Input: part model. Units: mm. Frame: model coordinates. Round coordinates to 2 decimals unless told otherwise and drop trailing zeros. Order: outer loops, then holes, each group sorted by start corner. A loop starts at its lowest first (then second) coordinate and runs counter-clockwise, first axis right, second up. Notation, with made-up numbers: (84.25, 51.5) -> (126.25, 51.5) arc R34 ccw to (126.25, 84.5) -> close; hole circle Ø10 at (-22.5, 49). An arc over 180 degrees is marked (long way). Use a Markdown table: item, result.
from build123d import *

# Parameters (mm, degrees)
SKETCH1_R           = 2.5
BOSS_EXTRUDE1_DEPTH = 5


with BuildPart() as part:
    # Sketch1 → Boss-Extrude1 (new body)
    with BuildSketch(Plane.XY):
        with BuildLine():
            Line((4.833962587, 7.00231299), (4.831156642, 7.163065475))
            Line((4.831156642, 7.163065475), (4.829008435, 7.286136175))
            Line((4.829008435, 7.286136175), (4.792643442, 9.369485213))
            Line((4.792643442, 9.369485213), (3.755980041, 9.831037496))
            Line((3.755980041, 9.831037496), (2.183417054, 8.464029347))
            Line((2.183417054, 8.464029347), (2.090520269, 8.383275404))
            Line((2.090520269, 8.383275404), (1.969180348, 8.27779622))
            ThreePointArc((1.969180348, 8.27779622), (1.769077823, 8.32285679), (1.567947285, 8.36308094))
            Line((1.567947285, 8.36308094), (1.5, 8.508794362))
            Line((1.5, 8.508794362), (1.447980152, 8.620351287))
            Line((1.447980152, 8.620351287), (0.567384684, 10.508794362))
            Line((0.567384684, 10.508794362), (-0.567384684, 10.508794362))
            Line((-0.567384684, 10.508794362), (-1.447980152, 8.620351287))
            Line((-1.447980152, 8.620351287), (-1.5, 8.508794362))
            Line((-1.5, 8.508794362), (-1.567947285, 8.36308094))
            ThreePointArc((-1.567947285, 8.36308094), (-1.769077823, 8.32285679), (-1.969180348, 8.27779622))
            Line((-1.969180348, 8.27779622), (-2.090520269, 8.383275404))
            Line((-2.090520269, 8.383275404), (-2.183417054, 8.464029347))
            Line((-2.183417054, 8.464029347), (-3.755980041, 9.831037496))
            Line((-3.755980041, 9.831037496), (-4.792643442, 9.369485213))
            Line((-4.792643442, 9.369485213), (-4.829008435, 7.286136175))
            Line((-4.829008435, 7.286136175), (-4.831156642, 7.163065475))
            Line((-4.831156642, 7.163065475), (-4.833962587, 7.00231299))
            ThreePointArc((-4.833962587, 7.00231299), (-5.001343841, 6.883759241), (-5.165818808, 6.761205332))
            Line((-5.165818808, 6.761205332), (-5.319570592, 6.808211969))
            Line((-5.319570592, 6.808211969), (-5.437281616, 6.844199841))
            Line((-5.437281616, 6.844199841), (-7.429901695, 7.453404935))
            Line((-7.429901695, 7.453404935), (-8.18921061, 6.610106952))
            Line((-8.18921061, 6.610106952), (-7.375057289, 4.692081926))
            Line((-7.375057289, 4.692081926), (-7.326962411, 4.578777493))
            Line((-7.326962411, 4.578777493), (-7.264141843, 4.430781509))
            ThreePointArc((-7.264141843, 4.430781509), (-7.368832073, 4.254397181), (-7.469240267, 4.075540618))
            Line((-7.469240267, 4.075540618), (-7.628818832, 4.055946834))
            Line((-7.628818832, 4.055946834), (-7.75099079, 4.040946004))
            Line((-7.75099079, 4.040946004), (-9.819125847, 3.787010949))
            Line((-9.819125847, 3.787010949), (-10.169788866, 2.707781148))
            Line((-10.169788866, 2.707781148), (-8.645891738, 1.286724086))
            Line((-8.645891738, 1.286724086), (-8.555869815, 1.202777285))
            Line((-8.555869815, 1.202777285), (-8.438284981, 1.093127654))
            ThreePointArc((-8.438284981, 1.093127654), (-8.462182296, 0.889411199), (-8.481162228, 0.685177906))
            Line((-8.481162228, 0.685177906), (-8.618974991, 0.602371644))
            Line((-8.618974991, 0.602371644), (-8.724483241, 0.538975892))
            Line((-8.724483241, 0.538975892), (-10.510533936, -0.534191634))
            Line((-10.510533936, -0.534191634), (-10.391918238, -1.662744616))
            Line((-10.391918238, -1.662744616), (-8.42177296, -2.341120038))
            Line((-8.42177296, -2.341120038), (-8.305389601, -2.381194042))
            Line((-8.305389601, -2.381194042), (-8.153371987, -2.433537904))
            ThreePointArc((-8.153371987, -2.433537904), (-8.092344324, -2.62936206), (-8.02661419, -2.82365829))
            Line((-8.02661419, -2.82365829), (-8.118832073, -2.955359075))
            Line((-8.118832073, -2.955359075), (-8.18943328, -3.056188048))
            Line((-8.18943328, -3.056188048), (-9.384575223, -4.763027631))
            Line((-9.384575223, -4.763027631), (-8.817190539, -5.745766731))
            Line((-8.817190539, -5.745766731), (-6.741453128, -5.564163239))
            Line((-6.741453128, -5.564163239), (-6.618832073, -5.553435287))
            Line((-6.618832073, -5.553435287), (-6.458666906, -5.53942265))
            ThreePointArc((-6.458666906, -5.53942265), (-6.323266501, -5.693494731), (-6.18419164, -5.844258315))
            Line((-6.18419164, -5.844258315), (-6.214869332, -6.002081362))
            Line((-6.214869332, -6.002081362), (-6.238355906, -6.12290931))
            Line((-6.238355906, -6.12290931), (-6.635938197, -8.16829288))
            Line((-6.635938197, -8.16829288), (-5.717890494, -8.835293579))
            Line((-5.717890494, -8.835293579), (-3.895474806, -7.825112067))
            Line((-3.895474806, -7.825112067), (-3.787818349, -7.765437119))
            Line((-3.787818349, -7.765437119), (-3.647199641, -7.687490896))
            ThreePointArc((-3.647199641, -7.687490896), (-3.460838455, -7.773170439), (-3.272466173, -7.854332985))
            Line((-3.272466173, -7.854332985), (-3.236299224, -8.010989254))
            Line((-3.236299224, -8.010989254), (-3.208610123, -8.130923927))
            Line((-3.208610123, -8.130923927), (-2.739887171, -10.161186083))
            Line((-2.739887171, -10.161186083), (-1.629915237, -10.397117901))
            Line((-1.629915237, -10.397117901), (-0.3759335, -8.73302793))
            Line((-0.3759335, -8.73302793), (-0.301856422, -8.634724327))
            Line((-0.301856422, -8.634724327), (-0.205098424, -8.506322127))
            ThreePointArc((-0.205098424, -8.506322127), (0, -8.508794362), (0.205098424, -8.506322127))
            Line((0.205098424, -8.506322127), (0.301856422, -8.634724327))
            Line((0.301856422, -8.634724327), (0.3759335, -8.73302793))
            Line((0.3759335, -8.73302793), (1.629915237, -10.397117901))
            Line((1.629915237, -10.397117901), (2.739887171, -10.161186083))
            Line((2.739887171, -10.161186083), (3.208610123, -8.130923927))
            Line((3.208610123, -8.130923927), (3.236299224, -8.010989254))
            Line((3.236299224, -8.010989254), (3.272466173, -7.854332985))
            ThreePointArc((3.272466173, -7.854332985), (3.460838455, -7.773170439), (3.647199641, -7.687490896))
            Line((3.647199641, -7.687490896), (3.787818349, -7.765437119))
            Line((3.787818349, -7.765437119), (3.895474806, -7.825112067))
            Line((3.895474806, -7.825112067), (5.717890494, -8.835293579))
            Line((5.717890494, -8.835293579), (6.635938197, -8.16829288))
            Line((6.635938197, -8.16829288), (6.238355906, -6.12290931))
            Line((6.238355906, -6.12290931), (6.214869332, -6.002081362))
            Line((6.214869332, -6.002081362), (6.18419164, -5.844258315))
            ThreePointArc((6.18419164, -5.844258315), (6.323266501, -5.693494731), (6.458666906, -5.53942265))
            Line((6.458666906, -5.53942265), (6.618832073, -5.553435287))
            Line((6.618832073, -5.553435287), (6.741453128, -5.564163239))
            Line((6.741453128, -5.564163239), (8.817190539, -5.745766731))
            Line((8.817190539, -5.745766731), (9.384575223, -4.763027631))
            Line((9.384575223, -4.763027631), (8.18943328, -3.056188048))
            Line((8.18943328, -3.056188048), (8.118832073, -2.955359075))
            Line((8.118832073, -2.955359075), (8.02661419, -2.82365829))
            ThreePointArc((8.02661419, -2.82365829), (8.092344324, -2.62936206), (8.153371987, -2.433537904))
            Line((8.153371987, -2.433537904), (8.305389601, -2.381194042))
            Line((8.305389601, -2.381194042), (8.42177296, -2.341120038))
            Line((8.42177296, -2.341120038), (10.391918238, -1.662744616))
            Line((10.391918238, -1.662744616), (10.510533936, -0.534191634))
            Line((10.510533936, -0.534191634), (8.724483241, 0.538975892))
            Line((8.724483241, 0.538975892), (8.618974991, 0.602371644))
            Line((8.618974991, 0.602371644), (8.481162228, 0.685177906))
            ThreePointArc((8.481162228, 0.685177906), (8.462182296, 0.889411199), (8.438284981, 1.093127654))
            Line((8.438284981, 1.093127654), (8.555869815, 1.202777285))
            Line((8.555869815, 1.202777285), (8.645891738, 1.286724086))
            Line((8.645891738, 1.286724086), (10.169788866, 2.707781148))
            Line((10.169788866, 2.707781148), (9.819125847, 3.787010949))
            Line((9.819125847, 3.787010949), (7.75099079, 4.040946004))
            Line((7.75099079, 4.040946004), (7.628818832, 4.055946834))
            Line((7.628818832, 4.055946834), (7.469240267, 4.075540618))
            ThreePointArc((7.469240267, 4.075540618), (7.368832073, 4.254397181), (7.264141843, 4.430781509))
            Line((7.264141843, 4.430781509), (7.326962411, 4.578777493))
            Line((7.326962411, 4.578777493), (7.375057289, 4.692081926))
            Line((7.375057289, 4.692081926), (8.18921061, 6.610106952))
            Line((8.18921061, 6.610106952), (7.429901695, 7.453404935))
            Line((7.429901695, 7.453404935), (5.437281616, 6.844199841))
            Line((5.437281616, 6.844199841), (5.319570592, 6.808211969))
            Line((5.319570592, 6.808211969), (5.165818808, 6.761205332))
            ThreePointArc((5.165818808, 6.761205332), (5.001343841, 6.883759241), (4.833962587, 7.00231299))
        make_face()
        Circle(SKETCH1_R, mode=Mode.SUBTRACT)
    extrude(amount=BOSS_EXTRUDE1_DEPTH)


solid = part.part
1) Draft query along Y for faces 1 (the face through (7.81, 7.03, 2.46)), 2 (the face through (-0.54, -2.44, 2.46)), 3 (the face through (2.18, -10.28, 2.46)), 4 (the face through (0, 3, 0)). Return one class per face: released by +Y, released by -Y, zero draft, split by the parting line, or undercut.
Answer key:
| item | result |
|---|---|
| face 1 | released by +Y |
| face 2 | undercut |
| face 3 | released by -Y |
| face 4 | zero draft |
2) Cut plane B-B on x = -7. Return loops of the section in (y, z).
Answer key:
| item | result |
|---|---|
| outline | (-5.59, 0) -> (7.32, 0) -> (7.32, 5) -> (-5.59, 5) -> close |
3) Cut plane C-C on y = 6. Return loops of the section in (x, z).
Answer key:
| item | result |
|---|---|
| outline | (-7.93, 0) -> (7.93, 0) -> (7.93, 5) -> (-7.93, 5) -> close |
4) Cut plane A-A on y = 0. Return loops of the section in (x, z).
Answer key:
| item | result |
|---|---|
| outline | (-9.62, 0) -> (-2.5, 0) -> (-2.5, 5) -> (-9.62, 5) -> close; (2.5, 0) -> (9.62, 0) -> (9.62, 5) -> (2.5, 5) -> close |
5) Contact query for flat-ended pins moving along their axis: P1, Ø3, axis at x = 1, z = 3, coming from the -Y side; P2, Ø2, axis at y = 0.5, z = 4, coming from the -X side. Output: stop coordinate, or through.
Answer key:
| item | result |
|---|---|
| P1 | stops at y = -10.4 |
| P2 | stops at x = -10.45 |
6) Ray query, probe 1 along X at (y, z) = (-8, 1); probe 2 along Y at (x, z) = (0, 3); probe 3 along Y at (x, z) = (-1, 1.9). Return the intervals inside material, ascending.
Answer key:
| item | result |
|---|---|
| probe 1 | x = -6.6 to -4.21, -3.24 to 3.24, 4.21 to 6.6 |
| probe 2 | y = -8.51 to -2.5, 2.5 to 10.51 |
| probe 3 | y = -9.56 to -2.29, 2.29 to 9.58 |
